The model under review builds one solid part; all positions refer to its coordinate system, in mm. Coordinates: 2 decimals unless noted, no trailing zeros. Order: outer loops, then holes, each group sorted by start corner. A loop starts at its lowest first (then second) coordinate and runs counter-clockwise, first axis right, second up. Notation, with made-up numbers: M 67,8 L 106,8 A11 cw 106,15 Z; hole C 35,52 d5. An arc over 180 degrees is marked long. Write each question's results on one line, items separated by ' | '.
from build123d import *

# Parameters (mm, degrees)
SKETCH1_R           = 15
SKETCH1_R_2         = 5
BOSS_EXTRUDE1_DEPTH = 5
SKETCH1_3_R         = 2.5
CUT_EXTRUDE1_DEPTH  = 5
CIRPATTERN1_COUNT   = 4
CHAMFER1_SIZE       = 1


with BuildPart() as part:
    # Sketch1 → Boss-Extrude1 (new body)
    with BuildSketch(Plane(origin=(0, 0, 0), x_dir=(1, 0, 0), z_dir=(0, 1, 0))):
        Circle(SKETCH1_R)
        Circle(SKETCH1_R_2, mode=Mode.SUBTRACT)
    extrude(amount=-BOSS_EXTRUDE1_DEPTH)

    # Sketch1_3 → Cut-Extrude1 (cut)
    with BuildSketch(Plane(origin=(0, 0, 0), x_dir=(1, 0, 0), z_dir=(0, 1, 0))):
        with Locations((0, 10)):
            Circle(SKETCH1_3_R)
    cut_extrude1 = extrude(amount=-CUT_EXTRUDE1_DEPTH, mode=Mode.SUBTRACT)

    # CirPattern1: Cut-Extrude1 ×4 about axis
    cirpattern1_axis = Axis((0, 0, 0), (0, 1, 0))
    for i in range(1, CIRPATTERN1_COUNT):
        add(cut_extrude1.rotate(cirpattern1_axis, i * 360 / CIRPATTERN1_COUNT), mode=Mode.SUBTRACT)

    # Chamfer1
    chamfer1_edges = [part.edges().sort_by_distance(p)[0] for p in [
        (-15, -5, 0),
    ]]
    chamfer(chamfer1_edges, length=CHAMFER1_SIZE)


solid = part.part
1) For pin 1 (2 mm diameter, centred on x = 9.5, y = -2.5, fed in from +Z); pin 2 (1.5 mm diameter, centred on x = -6, y = -1.5, fed in from +Z); pin 3 (1 mm diameter, centred on x = -8, y = -1.5, fed in from -Z), all flat-tipped, find the tip position at first contact; note any pin that passes through.
Solutions:
pin 1: z = 12.36 | pin 2: z = 14.05 | pin 3: z = -12.99
2) The part is to be moulded in two halves that separate along X. For faces 1 (the cylindrical face through (-7.56, -2.46, 0.54)), 2 (the flat face through (-4, 0, -4)), 3 (the cylindrical face through (-14.985, -1.972, -0.66)), say which applies: pulls with the +X half, pulls with the -X half, needs draft (parallel to the pull), parting line crosses it, or undercut.
Solutions:
face 1: undercut | face 2: needs draft | face 3: parting line crosses it
3) Take a section at C-C on y = -0.85. State the section outline as (x, z) points, plus the area to 3 significant figures.
Solutions:
outline: C 0,0 d30; hole C -10,0 d5; hole C 0,0 d10; hole C 0,-10 d5; hole C 0,10 d5; hole C 10,0 d5 | area: 550 mm2
4) Take a section at D-D on y = -4.4. State the section outline as (x, z) points.
Solutions:
outline: C 0,0 d29.2; hole C -10,0 d5; hole C 0,0 d10; hole C 0,-10 d5; hole C 0,10 d5; hole C 10,0 d5
5) To check wall thickness, follow line 1 along X through (y, z) = (-2.95, 0); line 2 along Z through (x, y) = (-1.5, -0.3). State the ranges of each line that lie inside material, in increasing order.
Solutions:
line 1: -15 to -12.5, -7.5 to -5, 5 to 7.5, 12.5 to 15 | line 2: -14.92 to -12, -8 to -4.77, 4.77 to 8, 12 to 14.92
6) Take a section at B-B on z = 0. State the section outline as (x, y) points.
Solutions:
outline: M -15,-4 L -14,-5 L -12.5,-5 L -12.5,0 L -15,0 Z; M -7.5,-5 L -5,-5 L -5,0 L -7.5,0 Z; M 5,-5 L 7.5,-5 L 7.5,0 L 5,0 Z; M 12.5,-5 L 14,-5 L 15,-4 L 15,0 L 12.5,0 Z
7) Take a section at A-A on x = 0. State the section outline as (y, z) points, plus the area to 3 significant figures.
Solutions:
outline: M -5,-14 L -4,-15 L 0,-15 L 0,-12.5 L -5,-12.5 Z; M -5,-7.5 L 0,-7.5 L 0,-5 L -5,-5 Z; M -5,5 L 0,5 L 0,7.5 L -5,7.5 Z; M -5,12.5 L 0,12.5 L 0,15 L -4,15 L -5,14 Z | area: 49.0 mm2
